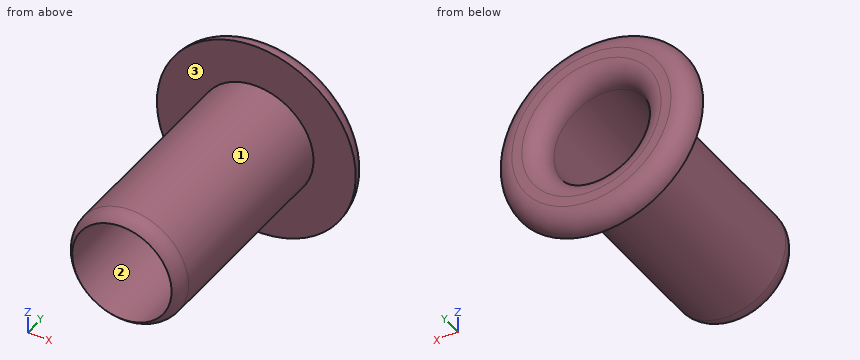
from build123d import *

# Parameters (mm, degrees)
SKETCH1_R           = 1.4605
BOSS_EXTRUDE1_DEPTH = 5.588
SKETCH2_R           = 2.54
BOSS_EXTRUDE2_DEPTH = 0.508
SKETCH3_R           = 1.27
CUT_EXTRUDE1_DEPTH  = 8.075621245
FILLET1_R           = 0.508


with BuildPart() as part:
    # Sketch1 → Boss-Extrude1 (new body)
    with BuildSketch(Plane(origin=(0, 0, 0), x_dir=(1, 0, 0), z_dir=(0, 1, 0))):
        with Locations(Location((0, 0, 0), (0, 0, 270))):
            Circle(SKETCH1_R)
    extrude(amount=BOSS_EXTRUDE1_DEPTH)

    # Sketch2 → Boss-Extrude2 (add)
    with BuildSketch(Plane(origin=(0, 5.588, 0), x_dir=(1, 0, 0), z_dir=(0, 1, 0))):
        with Locations(Location((0, 0, 0), (0, 0, 270))):
            Circle(SKETCH2_R)
    extrude(amount=BOSS_EXTRUDE2_DEPTH)

    # Sketch3 → Cut-Extrude1 (cut, through all)
    with BuildSketch(Plane(origin=(0, 6.096, 0), x_dir=(1, 0, 0), z_dir=(0, 1, 0))):
        with Locations(Location((0, 0, 0), (0, 0, 270))):
            Circle(SKETCH3_R)
    extrude(amount=-CUT_EXTRUDE1_DEPTH, mode=Mode.SUBTRACT)

    # Fillet1
    # the kernel refuses this fillet: 0.508 mm, written as the material it takes off along each edge
    with BuildSketch(Plane(origin=(0, 6.096, 0), x_dir=(0, 0, 1), z_dir=(-1, 0, 0))) as fillet1_piece_1:
        with BuildLine():
            CenterArc((1.27 + FILLET1_R, -FILLET1_R), FILLET1_R, 90, 90)
            Line((1.27, -FILLET1_R), (1.27 - FILLET1_R * 0.02, -FILLET1_R))
            Line((1.27 - FILLET1_R * 0.02, -FILLET1_R), (1.27 - FILLET1_R * 0.02, FILLET1_R * 0.02))
            Line((1.27 - FILLET1_R * 0.02, FILLET1_R * 0.02), (1.27 + FILLET1_R, FILLET1_R * 0.02))
            Line((1.27 + FILLET1_R, FILLET1_R * 0.02), (1.27 + FILLET1_R, 0))
        make_face()
    revolve(axis=Axis((0, 6.096, 0), (0, 1, 0)), mode=Mode.SUBTRACT)
    with BuildSketch(Plane(origin=(0, 0, 0), x_dir=(0, 0, 1), z_dir=(-1, 0, 0))) as fillet1_piece_2:
        with BuildLine():
            CenterArc((0.9525, 0.396557373), FILLET1_R, 308.682187453, 51.317812547)
            Line((1.27, 0), (1.27635, -0.007931147))
            ThreePointArc((1.27635, -0.007931147), (1.36525, -0.01016), (1.4605, -0.01016))
            Line((1.4605, -0.01016), (1.47066, 0))
            Line((1.47066, 0), (1.47066, 0.396557373))
            Line((1.47066, 0.396557373), (1.4605, 0.396557373))
        make_face()
    revolve(axis=Axis((0, 0, 0), (0, 1, 0)), mode=Mode.SUBTRACT)
    with BuildSketch(Plane(origin=(0, 6.096, 0), x_dir=(0, 0, 1), z_dir=(-1, 0, 0))) as fillet1_piece_3:
        with BuildLine():
            CenterArc((2.54 - FILLET1_R, -FILLET1_R), FILLET1_R, 0, 90)
            Line((2.54 - FILLET1_R, 0), (2.54 - FILLET1_R, FILLET1_R * 0.02))
            Line((2.54 - FILLET1_R, FILLET1_R * 0.02), (2.54 + FILLET1_R * 0.02, FILLET1_R * 0.02))
            Line((2.54 + FILLET1_R * 0.02, FILLET1_R * 0.02), (2.54 + FILLET1_R * 0.02, -FILLET1_R))
            Line((2.54 + FILLET1_R * 0.02, -FILLET1_R), (2.54, -FILLET1_R))
        make_face()
    revolve(axis=Axis((0, 6.096, 0), (0, 1, 0)), mode=Mode.SUBTRACT)


solid = part.part
Model file for the job. Use its own axes, mm. Face numbers are marked on the shaded views. Give positions to 0.01 mm unless a question says otherwise; leave off trailing zeros. Write each loop counter-clockwise with the first axis right and the second up, starting at its lowest first coordinate (ties: lowest second). Pieces come first, ordered by that corner, then holes. Notation, with made-up numbers: (67.25, 79) -> (83.25, 79) arc R25 ccw to (83.25, 94) -> close; hole circle Ø1 at (-14.75, 32.5). An arc over 180 degrees is marked (long way). Write item = value, one per line.
(1) Slice it at D-D, the plane y = 5.75. Give the cut face in (x, z), then the cut area to 3 significant figures.
Determined:
outline = circle Ø5.03 at (0, 0); hole circle Ø2.59 at (0, 0)
area = 14.6 mm2
(2) Probe line 1 along X through (y, z) = (3.4, 0); line 2 along X through (y, z) = (5.5, -0.65); line 3 along Z through (x, y) = (-1, 0.5). List the from-to ranges inside material, lowest first.
Determined:
line_1 = -1.46 to -1.27, 1.27 to 1.46
line_2 = -1.31 to -1.09, 1.09 to 1.31
line_3 = -1.06 to -0.78, 0.78 to 1.06
(3) Slice it at B-B, the plane x = 0. Give the cut face in (y, z).
Determined:
outline = (0, -1.27) arc R0.51 ccw to (0.4, -1.46) -> (5.59, -1.46) -> (5.59, -2.54) arc R0.51 ccw to (6.1, -2.03) -> (6.1, -1.78) arc R0.51 ccw to (5.59, -1.27) -> close; (0, 1.27) -> (5.59, 1.27) arc R0.51 ccw to (6.1, 1.78) -> (6.1, 2.03) arc R0.51 ccw to (5.59, 2.54) -> (5.59, 1.46) -> (0.4, 1.46) arc R0.51 ccw to start
(4) Slice it at A-A, the plane z = 0. Give the cut face in (x, y), then the cut area to 3 significant figures.
Determined:
outline = (-2.54, 5.59) -> (-1.46, 5.59) -> (-1.46, 0.4) arc R0.51 ccw to (-1.27, 0) -> (-1.27, 5.59) arc R0.51 ccw to (-1.78, 6.1) -> (-2.03, 6.1) arc R0.51 ccw to start; (1.27, 0) arc R0.51 ccw to (1.46, 0.4) -> (1.46, 5.59) -> (2.54, 5.59) arc R0.51 ccw to (2.03, 6.1) -> (1.78, 6.1) arc R0.51 ccw to (1.27, 5.59) -> close
area = 3.15 mm2
(5) Slice it at C-C, the plane y = 3. Give the cut face in (x, z).
Determined:
outline = circle Ø2.92 at (0, 0); hole circle Ø2.54 at (0, 0)
(6) Mould opens along Z. For the marked faces 1, 2 and 3 say: released by +Z, released by -Z, zero draft, split by the parting line, or undercut.
Determined:
face_1 = split by the parting line
face_2 = undercut
face_3 = zero draft
(7) Flat gauge pin, fed straight in: P1, Ø2, axis at x = -0.5, y = 2, coming from the +Z side. Where does the tip first touch, or does it go through?
Determined:
P1 = 1.46
